Design review of the part built by this model. Coordinates are the model's own, in mm. A direction names the side the tool comes from. Give positions to 0.01 mm unless a question says otherwise; leave off trailing zeros. Order: outer loops, then holes, each group sorted by start corner. A loop starts at its lowest first (then second) coordinate and runs counter-clockwise, first axis right, second up. Notation, with made-up numbers: (33, 73) -> (56, 73) arc R30 cw to (56, 99) -> close; hole circle Ø4 at (15.5, -35). An arc over 180 degrees is marked (long way). One line per item, written item: value.
from build123d import *

# Parameters (mm, degrees)
BOSS_EXTRUDE2_DEPTH     = 15
SKETCH1_6_R             = 25
BOSS_EXTRUDE3_DEPTH     = 30
SKETCH1_7_R             = 32.5
BOSS_EXTRUDE4_DEPTH     = 40
BOSS_EXTRUDE5_DEPTH     = 20
SHELL1_T                = -5
RIB1_START              = -5
RIB1_DEPTH              = 10
CIRPATTERN1_COUNT       = 3
CUT_EXTRUDE1_DEPTH      = 144.713620755
CUT_EXTRUDE1_DEPTH_BACK = 144.713620755
SKETCH1_8_R             = 10
SKETCH1_8_R_2           = 9.896657658
KEYWAY_DEPTH            = 161.809545085


# Read off the part's stored shape, not the designer's step: Rib1
with BuildPart() as part:
    # Sketch1 → Boss-Extrude2 (new body)
    with BuildSketch(Plane.XY):
        with BuildLine():
            ThreePointArc((24.536591615, 79.791207774), (0, 100), (-24.536591615, 79.791207774))
            ThreePointArc((-24.536591615, 79.791207774), (-44.738287256, 25.82966219), (-81.369508738, -18.646292226))
            ThreePointArc((-81.369508738, -18.646292226), (-86.602540378, -50), (-56.832917123, -61.144915548))
            ThreePointArc((-56.832917123, -61.144915548), (0, -51.65932438), (56.832917123, -61.144915548))
            ThreePointArc((56.832917123, -61.144915548), (86.602540378, -50), (81.369508738, -18.646292226))
            ThreePointArc((81.369508738, -18.646292226), (44.738287256, 25.82966219), (24.536591615, 79.791207774))
        make_face()
    extrude(amount=BOSS_EXTRUDE2_DEPTH)

    # Sketch1<6> → Boss-Extrude3 (add)
    with BuildSketch(Plane.XY):
        with Locations(Location((0, 75, 0), (0, 0, 168.951006611))):
            Circle(SKETCH1_6_R)
        with Locations(Location((64.951905284, -37.5, 0), (0, 0, 251.048993389))):
            Circle(SKETCH1_6_R)
        with Locations(Location((-64.951905284, -37.5, 0), (0, 0, 131.048993389))):
            Circle(SKETCH1_6_R)
    extrude(amount=BOSS_EXTRUDE3_DEPTH)

    # Sketch1<7> → Boss-Extrude4 (add)
    with BuildSketch(Plane.XY):
        Circle(SKETCH1_7_R)
    extrude(amount=BOSS_EXTRUDE4_DEPTH)


with BuildPart() as body_2:
    # Sketch2 → Boss-Extrude5 (new body)
    with BuildSketch(Plane(origin=(0, 0, 0), x_dir=(-1, 0, 0), z_dir=(0, 0, -1))):
        with BuildLine():
            Line((-88.767603888, -23.75), (-23.815698604, 88.75))
            ThreePointArc((-23.815698604, 88.75), (0, 102.5), (23.815698604, 88.75))
            Line((23.815698604, 88.75), (88.767603888, -23.75))
            ThreePointArc((88.767603888, -23.75), (88.767603888, -51.25), (64.951905284, -65))
            Line((64.951905284, -65), (-64.951905284, -65))
            ThreePointArc((-64.951905284, -65), (-88.767603888, -51.25), (-88.767603888, -23.75))
        make_face()
    extrude(amount=BOSS_EXTRUDE5_DEPTH)

    # Shell1
    shell1_openings = [body_2.faces().sort_by_distance(p)[0] for p in [
        (0, 0, -20),
    ]]
    offset(amount=SHELL1_T, openings=shell1_openings, kind=Kind.INTERSECTION)

    # Combine1: union part
    add(part.part)

    # Rib1 outline → Rib1 (add)
    with BuildSketch(Plane(origin=(0, 0, 0), x_dir=(0, 0, -1), z_dir=(1, 0, 0)).offset(RIB1_START)):
        Polygon((-27.5, 52), (-27.5, 43.5), (-32.67587207, 32.113081447), (-33.181818182, 31), (-15, 31), (-15, 52), align=None)
    rib1 = extrude(amount=RIB1_DEPTH)

    # CirPattern1: Rib1 ×3 about axis
    cirpattern1_axis = Axis((0, 0, 0), (0, 0, 1))
    for i in range(1, CIRPATTERN1_COUNT):
        add(rib1.rotate(cirpattern1_axis, i * 360 / CIRPATTERN1_COUNT))

    # Sketch1<8> → Cut-Extrude1 (cut, two sides: drawn at the far end of the back side and taken through both)
    with BuildSketch(Plane.XY.offset(-CUT_EXTRUDE1_DEPTH_BACK)):
        with Locations((0, 75)):
            Circle(SKETCH1_8_R)
        with Locations((-64.951905284, -37.5)):
            Circle(SKETCH1_8_R)
        with Locations((64.951905284, -37.5)):
            Circle(SKETCH1_8_R_2)
    extrude(amount=CUT_EXTRUDE1_DEPTH + CUT_EXTRUDE1_DEPTH_BACK, mode=Mode.SUBTRACT)

    # KeySketch → Keyway (cut, through all)
    with BuildSketch(Plane(origin=(-6.035211163, -9.571395477, 40), x_dir=(1, 0, 0), z_dir=(0, 0, 1))):
        with BuildLine():
            Line((12.035211163, -9.507388551), (12.035211163, -13.728604523))
            Line((12.035211163, -13.728604523), (0.035211163, -13.728604523))
            Line((0.035211163, -13.728604523), (0.035211163, -9.507388551))
            ThreePointArc((0.035211163, -9.507388551), (6.035211163, 29.571395477), (12.035211163, -9.507388551))
        make_face()
    extrude(amount=-KEYWAY_DEPTH, mode=Mode.SUBTRACT)


solid = body_2.part
Item 1: Add section C-C on z = 21.5. Give the boundary of the cut face in (x, y), plus the area to 3 significant figures.
Returned:
outline: (-46.24, -20.92) arc R25 ccw (long way) to (-41.24, -29.58) -> (-25.31, -20.39) arc R32.5 ccw to (25.31, -20.39) -> (41.24, -29.58) arc R25 ccw (long way) to (46.24, -20.92) -> (30.31, -11.73) arc R32.5 ccw to (5, 32.11) -> (5, 50.51) arc R25 ccw (long way) to (-5, 50.51) -> (-5, 32.11) arc R32.5 ccw to (-30.31, -11.73) -> close; hole circle Ø20 at (-64.95, -37.5); hole circle Ø20 at (0, 75); hole (-6, -23.3) -> (6, -23.3) -> (6, -19.08) arc R20 ccw (long way) to (-6, -19.08) -> close; hole circle Ø19.79 at (64.95, -37.5)
area: 7,510 mm²
Item 2: Add section A-A on x = 0. Give the boundary of the cut face in (y, z).
Returned:
outline: (-65, -20) -> (-60, -20) -> (-60, -5) -> (-23.3, -5) -> (-23.3, 40) -> (-32.5, 40) -> (-32.5, 15) -> (-51.66, 15) -> (-51.66, 0) -> (-65, 0) -> close; (20, -5) -> (65, -5) -> (65, 30) -> (50, 30) -> (50, 27.5) -> (43.5, 27.5) -> (32.5, 32.5) -> (32.5, 40) -> (20, 40) -> close; (85, -5) -> (97.5, -5) -> (97.5, -20) -> (102.5, -20) -> (102.5, 0) -> (100, 0) -> (100, 30) -> (85, 30) -> close
Item 3: Machinability: for faces 1 (the flat face through (52.416, 29.213, -12.395)), 2 (the flat face through (5, 41, 22)), 3 (the cylindrical face through (31, 9.76, 27.32)), which of the approach directions +Z, -Z, +X, -X, +Y, -Y give a long, thin tool a straight path to every point of the face, cutting with its end or side? Answer none if there is none.
Returned:
face 1: -Z
face 2: +Z, +X
face 3: +Z
Item 4: Clearance check with flat-ended pins moving along their axes: P1, Ø7.5, axis at x = 25, z = -14.5, coming from the +Y side; P2, Ø12, axis at x = 64.95, y = -37.5, coming from the +Z side; P3, Ø3.5, axis at y = -21, z = 16, coming from the -X side; P4, Ø10, axis at y = 58, z = 4.5, coming from the -X side. State where each tip first meets the part, or that it passes through.
Returned:
P1: y = 92.46
P2: through
P3: x = -85.14
P4: x = -42.83
Item 5: Add section B-B on y = -37.5. Give the boundary of the cut face in (x, z).
Returned:
outline: (-92.45, -20) -> (-87.45, -20) -> (-87.45, -5) -> (-74.95, -5) -> (-74.95, 30) -> (-89.95, 30) -> (-89.95, 0) -> (-92.45, 0) -> close; (-54.95, -5) -> (55.06, -5) -> (55.06, 30) -> (39.95, 30) -> (39.95, 15) -> (-39.95, 15) -> (-39.95, 30) -> (-54.95, 30) -> close; (74.85, -5) -> (87.45, -5) -> (87.45, -20) -> (92.45, -20) -> (92.45, 0) -> (89.95, 0) -> (89.95, 30) -> (74.85, 30) -> close
Item 6: To check wall thickness, follow line 1 along X through (y, z) = (-37, 12); line 2 along X through (y, z) = (-37.5, 7); line 3 along Y through (x, z) = (-65, 29). State the ranges of each line that lie inside material, in increasing order. Write a range as from..to.
Returned:
line 1: -89.95..-74.94, -54.96..55.07, 74.84..89.95
line 2: -89.95..-74.95, -54.95..55.06, 74.85..89.95
line 3: -62.5..-47.5, -27.5..-12.5
Item 7: Add section D-D on y = -3.5. Give the boundary of the cut face in (x, z), plus the area to 3 significant figures.
Returned:
outline: (-77.08, -20) -> (-71.3, -20) -> (-71.3, -5) -> (-19.69, -5) -> (-19.69, 40) -> (-32.31, 40) -> (-32.31, 15) -> (-66, 15) -> (-66, 0) -> (-77.08, 0) -> close; (19.69, -5) -> (71.3, -5) -> (71.3, -20) -> (77.08, -20) -> (77.08, 0) -> (66, 0) -> (66, 15) -> (32.31, 15) -> (32.31, 40) -> (19.69, 40) -> close
area: 2,770 mm²
